```python
from build123d import *

# Parameters (mm, degrees)
SKETCH1_R           = 1.75
BOSS_EXTRUDE1_DEPTH = 4
BOSS_EXTRUDE3_START = -4
BOSS_EXTRUDE3_DEPTH = 4
SKETCH4_R           = 1.3
SKETCH4_R_2         = 2.4
CUT_EXTRUDE1_DEPTH  = 4


with BuildPart() as part:
    # Sketch1 → Boss-Extrude1 (new body)
    with BuildSketch(Plane(origin=(0, 0, 0), x_dir=(1, 0, 0), z_dir=(0, 1, 0))):
        with BuildLine():
            Line((30.75, 4), (11.409123542, 4))
            ThreePointArc((11.409123542, 4), (-12.09, 0), (11.409123542, -4))
            Line((11.409123542, -4), (30.75, -4))
            ThreePointArc((30.75, -4), (34.75, 0), (30.75, 4))
        make_face()
        with Locations(Location((30.75, 0, 0), (0, 0, 270))):
            Circle(SKETCH1_R, mode=Mode.SUBTRACT)
        with Locations(Location((0, 0, 0), (0, 0, 270))):
            Circle(SKETCH1_R, mode=Mode.SUBTRACT)
    extrude(amount=BOSS_EXTRUDE1_DEPTH)

    # Sketch3 → Boss-Extrude3 (add)
    with BuildSketch(Plane(origin=(0, 4, 0), x_dir=(1, 0, 0), z_dir=(0, 1, 0)).offset(BOSS_EXTRUDE3_START)):
        with BuildLine():
            ThreePointArc((12.82210701, 7.044889767), (12.669951657, 7.315), (12.51210701, 7.581825517))
            ThreePointArc((12.51210701, 7.581825517), (11.170223244, 7.416617696), (9.911436862, 6.9232593))
            ThreePointArc((9.911436862, 6.9232593), (10.470247132, 6.045), (10.951436862, 5.12192646))
            ThreePointArc((10.951436862, 5.12192646), (12.008090957, 5.965388247), (12.82210701, 7.044889767))
        make_face()
        with BuildLine():
            ThreePointArc((-14.626715284, 0.31), (-13.382005944, 0.837867713), (-12.04518576, 1.04))
            ThreePointArc((-12.04518576, 1.04), (-12.09, 0), (-12.04518576, -1.04))
            ThreePointArc((-12.04518576, -1.04), (-13.382005944, -0.837867713), (-14.626715284, -0.31))
            ThreePointArc((-14.626715284, -0.31), (-14.63, 0), (-14.626715284, 0.31))
        make_face()
        with BuildLine():
            ThreePointArc((-14.048088143, 4.085109489), (-12.709169027, 4.272836063), (-11.365584201, 4.122086336))
            ThreePointArc((-11.365584201, 4.122086336), (-11.67804324, 3.129122255), (-11.903927815, 2.112960617))
            ThreePointArc((-11.903927815, 2.112960617), (-13.14288127, 2.654199937), (-14.208555951, 3.486235477))
            ThreePointArc((-14.208555951, 3.486235477), (-14.131494839, 3.78652263), (-14.048088143, 4.085109489))
        make_face()
        with BuildLine():
            ThreePointArc((-12.51210701, 7.581825517), (-11.170223244, 7.416617696), (-9.911436862, 6.9232593))
            ThreePointArc((-9.911436862, 6.9232593), (-10.470247132, 6.045), (-10.951436862, 5.12192646))
            ThreePointArc((-10.951436862, 5.12192646), (-12.008090957, 5.965388247), (-12.82210701, 7.044889767))
            ThreePointArc((-12.82210701, 7.044889767), (-12.669951657, 7.315), (-12.51210701, 7.581825517))
        make_face()
        with BuildLine():
            ThreePointArc((-10.123446462, 10.561852666), (-8.870045207, 10.05496909), (-7.781841479, 9.252623584))
            ThreePointArc((-7.781841479, 9.252623584), (-8.548920985, 8.548920985), (-9.252623584, 7.781841479))
            ThreePointArc((-9.252623584, 7.781841479), (-10.05496909, 8.870045207), (-10.561852666, 10.123446462))
            ThreePointArc((-10.561852666, 10.123446462), (-10.344972209, 10.344972209), (-10.123446462, 10.561852666))
        make_face()
        with BuildLine():
            ThreePointArc((-7.044889767, 12.82210701), (-5.965388247, 12.008090957), (-5.12192646, 10.951436862))
            ThreePointArc((-5.12192646, 10.951436862), (-6.045, 10.470247132), (-6.9232593, 9.911436862))
            ThreePointArc((-6.9232593, 9.911436862), (-7.416617696, 11.170223244), (-7.581825517, 12.51210701))
            ThreePointArc((-7.581825517, 12.51210701), (-7.315, 12.669951657), (-7.044889767, 12.82210701))
        make_face()
        with BuildLine():
            ThreePointArc((-3.486235477, 14.208555951), (-2.654199937, 13.14288127), (-2.112960617, 11.903927815))
            ThreePointArc((-2.112960617, 11.903927815), (-3.129122255, 11.67804324), (-4.122086336, 11.365584201))
            ThreePointArc((-4.122086336, 11.365584201), (-4.272836063, 12.709169027), (-4.085109489, 14.048088143))
            ThreePointArc((-4.085109489, 14.048088143), (-3.78652263, 14.131494839), (-3.486235477, 14.208555951))
        make_face()
        with BuildLine():
            ThreePointArc((0.31, 14.626715284), (0.837867713, 13.382005944), (1.04, 12.04518576))
            ThreePointArc((1.04, 12.04518576), (0, 12.09), (-1.04, 12.04518576))
            ThreePointArc((-1.04, 12.04518576), (-0.837867713, 13.382005944), (-0.31, 14.626715284))
            ThreePointArc((-0.31, 14.626715284), (0, 14.63), (0.31, 14.626715284))
        make_face()
        with BuildLine():
            ThreePointArc((4.085109489, 14.048088143), (4.272836063, 12.709169027), (4.122086336, 11.365584201))
            ThreePointArc((4.122086336, 11.365584201), (3.129122255, 11.67804324), (2.112960617, 11.903927815))
            ThreePointArc((2.112960617, 11.903927815), (2.654199937, 13.14288127), (3.486235477, 14.208555951))
            ThreePointArc((3.486235477, 14.208555951), (3.78652263, 14.131494839), (4.085109489, 14.048088143))
        make_face()
        with BuildLine():
            ThreePointArc((7.581825517, 12.51210701), (7.416617696, 11.170223244), (6.9232593, 9.911436862))
            ThreePointArc((6.9232593, 9.911436862), (6.045, 10.470247132), (5.12192646, 10.951436862))
            ThreePointArc((5.12192646, 10.951436862), (5.965388247, 12.008090957), (7.044889767, 12.82210701))
            ThreePointArc((7.044889767, 12.82210701), (7.315, 12.669951657), (7.581825517, 12.51210701))
        make_face()
        with BuildLine():
            ThreePointArc((10.561852666, 10.123446462), (10.05496909, 8.870045207), (9.252623584, 7.781841479))
            ThreePointArc((9.252623584, 7.781841479), (8.548920985, 8.548920985), (7.781841479, 9.252623584))
            ThreePointArc((7.781841479, 9.252623584), (8.870045207, 10.05496909), (10.123446462, 10.561852666))
            ThreePointArc((10.123446462, 10.561852666), (10.344972209, 10.344972209), (10.561852666, 10.123446462))
        make_face()
    extrude(amount=BOSS_EXTRUDE3_DEPTH)

    # Sketch4 → Cut-Extrude1 (cut)
    with BuildSketch(Plane(origin=(0, 4, 0), x_dir=(1, 0, 0), z_dir=(0, 1, 0))):
        with Locations(Location((4.5, 0.592436239, 0), (0, 0, 270))):
            Circle(SKETCH4_R)
        with Locations(Location((-4.5, -0.592436239, 0), (0, 0, 270))):
            Circle(SKETCH4_R)
        with Locations(Location((0, 0, 0), (0, 0, 270))):
            Circle(SKETCH4_R_2)
    extrude(amount=-CUT_EXTRUDE1_DEPTH, mode=Mode.SUBTRACT)


solid = part.part
```
Verification items for the finished model (mm, model axes). A direction names the side the tool comes from. Give positions to 0.01 mm unless a question says otherwise; leave off trailing zeros. Order: outer loops, then holes, each group sorted by start corner. A loop starts at its lowest first (then second) coordinate and runs counter-clockwise, first axis right, second up. Notation, with made-up numbers: M -18,86.25 L 25,86.25 A18 ccw 25,100.25 Z; hole C -32,5.25 d1. An arc over 180 degrees is marked long. Return JSON: item names as keys, results as strings. Group by question number.
1) Mould release check, pull along Z, two halves, no side actions. Record for faces 6 (the face through (1.586, 1.972, -11.986)), 7 (the face through (-4.273, 1.972, -12.69)), 8 (the face through (4, 0, 2)): pulls with the +Z half, pulls with the -Z half, needs draft (parallel to the pull), parting line crosses it, or undercut.
2) Section check C-C on z = 10.25. Record the cut outline in (x, y).
3) Section check A-A on y = 1.55. Give the number of separate pieces and of enclosed holes in the cut face, and give its area (3 significant figures).
4) Section check B-B on x = 16. Record the cut outline in (y, z).
5) Access from +Z, -Z, +X, -X, +Y, -Y to the whole of each face (thin tool, end or side, straight path). Record for faces 1 (the face through (0.833, 1.972, -13.4)), 2 (the face through (10.064, 1.972, -8.887)), 3 (the face through (-1.742, 1.972, 11.964)), 4 (the face through (7.366, 1.972, -9.587)), 5 (the face through (-13.4, 1.972, -0.833)).
6) Go/stop test with flat-tipped pins: pin 1 Ø1.5 at (y, z) = (1.5, 5.5) entering from +X; pin 2 Ø1.2 at (x, y) = (24.5, 2) entering from +Z. Record where each tip stops, or that it passes through.
7) Scan lines: line 1 (X direction, y = 1.8, z = -11.5); line 2 (X direction, y = 1.3, z = 0); line 3 (X direction, y = 1.95, z = -12.5). Record each from-to range of solid material in increasing order.
Answer block:
{
 "1": {"face 6": "pulls with the -Z half", "face 7": "undercut", "face 8": "needs draft"},
 "2": {"outline": "M -6.41,0 L 6.41,0 L 6.41,4 L -6.41,4 Z"},
 "3": {"separate pieces": "1", "enclosed holes": "4", "area": "641 mm^2"},
 "4": {"outline": "M 0,-4 L 4,-4 L 4,4 L 0,4 Z"},
 "5": {"face 1": "-Z, +Y, -Y", "face 2": "+X, +Y, -Y", "face 3": "+Z, +Y, -Y", "face 4": "+Y, -Y", "face 5": "-X, +Y, -Y"},
 "6": {"pin 1": "stops at x = 11.12", "pin 2": "stops at z = 4"},
 "7": {"line 1": "x = -7.49 to -5.51, -4.15 to 4.15, 5.51 to 7.49", "line 2": "x = -14.63 to -5.66, -3.34 to -2.4, 2.4 to 3.34, 5.66 to 29, 32.5 to 34.75", "line 3": "x = -7.58 to -6.55, -4.27 to -2.33, -1.01 to 1.01, 2.33 to 4.27, 6.55 to 7.58"}
}
